Can you work these out from the model? Positions are in its coordinate system, mm. Face numbers are marked on the shaded views. A direction names the side the tool comes from. Coordinates: 2 decimals unless noted, no trailing zeros. Order: outer loops, then holes, each group sorted by start corner. A loop starts at its lowest first (then second) coordinate and runs counter-clockwise, first axis right, second up. Notation, with made-up numbers: M 67.25,-13.75 L 97.25,-13.75 A18 cw 97.25,-7.75 Z; hole C -12,41 d4. An arc over 180 degrees is marked long. Answer as a JSON object with one key per item and string values.
from build123d import *

# Parameters (mm, degrees)
F0_W      = 60
F0_H      = 60
F0_R      = 2.3
F0_R_2    = 19.05
F0_R_3    = 4
F1_DEPTH  = 4.8
F2_DEPTH  = 1.6
F3_DEPTH  = 20.6
F4_R      = 4
F5_W      = 15
F5_H      = 0.5
F6_DEPTH  = 60.001
F7_W      = 37.14
F7_H      = 11.43
F7_H_2    = 37.14
F7_W_2    = 11.43
F8_DEPTH  = 89
F9_R      = 4
F10_R     = 3
F11_R     = 3.25
F12_DEPTH = 14


with BuildPart() as f1:
    # F0 (on Front) → F1 (new body)
    with BuildSketch(Plane.XZ):
        Rectangle(F0_W, F0_H)
        with Locations((-25.1, -25.1)):
            Circle(F0_R, mode=Mode.SUBTRACT)
        with Locations((25.1, -25.1)):
            Circle(F0_R, mode=Mode.SUBTRACT)
        with Locations((-25.1, 25.1)):
            Circle(F0_R, mode=Mode.SUBTRACT)
        Circle(F0_R_2, mode=Mode.SUBTRACT)
        with Locations((25.1, 25.1)):
            Circle(F0_R, mode=Mode.SUBTRACT)
        Circle(F0_R_2)
        Circle(F0_R_3, mode=Mode.SUBTRACT)
        Circle(F0_R_3)
    extrude(amount=-F1_DEPTH)

    # F0 (on Front) → F2 (join)
    with BuildSketch(Plane.XZ):
        Circle(F0_R_2)
        Circle(F0_R_3, mode=Mode.SUBTRACT)
    extrude(amount=F2_DEPTH)

    # F0 (on Front) → F3 (join)
    with BuildSketch(Plane.XZ):
        Circle(F0_R_3)
    extrude(amount=F3_DEPTH)

    # F4
    f4_edges = [f1.edges().sort_by_distance(p)[0] for p in [
        (-30, 2.4, 30),
        (30, 2.4, 30),
        (30, 2.4, -30),
        (-30, 2.4, -30),
    ]]
    fillet(f4_edges, radius=F4_R)

    # F5 (on face) → F6 (cut, through all)
    with BuildSketch(Plane(origin=(-30, 0, 0), x_dir=(0, -1, 0), z_dir=(-1, 0, 0))):
        with Locations((13.1, 3.75)):
            Rectangle(F5_W, F5_H)
    extrude(amount=-F6_DEPTH, mode=Mode.SUBTRACT)

    # F7 (on Front) → F8 (join)
    with BuildSketch(Plane.XZ):
        with Locations((0, 24.285)):
            Rectangle(F7_W, F7_H)
        Rectangle(F7_W, F7_H_2)
        with Locations((-24.285, 0)):
            Rectangle(F7_W_2, F7_H_2)
        with Locations((24.285, 0)):
            Rectangle(F7_W_2, F7_H_2)
        with Locations((0, -24.285)):
            Rectangle(F7_W, F7_H)
    extrude(amount=-F8_DEPTH)

    # F9
    f9_edges = [f1.edges().sort_by_distance(p)[0] for p in [
        (18.57, 46.9, 18.57),
        (-18.57, 46.9, 18.57),
        (-18.57, 46.9, -18.57),
        (18.57, 46.9, -18.57),
    ]]
    fillet(f9_edges, radius=F9_R)

    # F10
    f10_edges = [f1.edges().sort_by_distance(p)[0] for p in [
        (18.57, 46.9, 30),
        (30, 46.9, 18.57),
        (30, 46.9, -18.57),
        (18.57, 46.9, -30),
        (-18.57, 46.9, -30),
        (-30, 46.9, -18.57),
        (-30, 46.9, 18.57),
        (-18.57, 46.9, 30),
    ]]
    fillet(f10_edges, radius=F10_R)

    # F11 (on face) → F12 (join)
    with BuildSketch(Plane(origin=(0, 89, 0), x_dir=(-1, 0, 0), z_dir=(0, 1, 0))):
        Circle(F11_R)
    extrude(amount=F12_DEPTH)


solid = f1.part
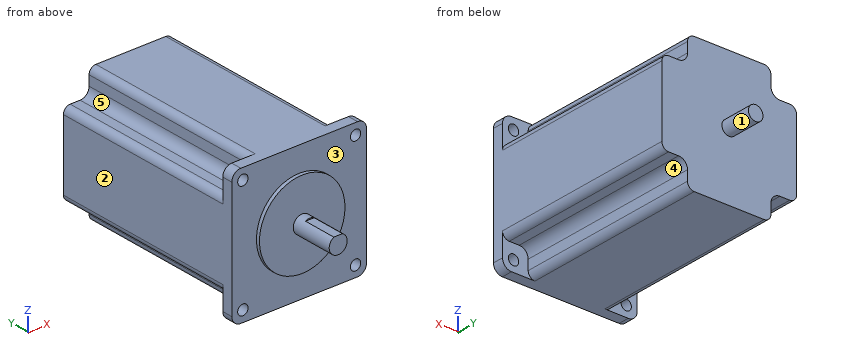
Item 1: I want a section at A-A, the plane x = 0. Write out the boundary of the cut face in (y, z), plus the area to 3 significant figures.
Answers follow:
{"outline": "M -20.6,-4 L -1.6,-4 L -1.6,-19.05 L 0,-19.05 L 0,-30 L 89,-30 L 89,-3.25 L 103,-3.25 L 103,3.25 L 89,3.25 L 89,30 L 0,30 L 0,19.05 L -1.6,19.05 L -1.6,4 L -5.6,4 L -5.6,3.5 L -20.6,3.5 Z", "area": "5,640 mm^2"}
Item 2: I want a section at B-B, the plane y = 53.5. Write out the boundary of the cut face in (x, z), plus the area to 3 significant figures.
Answers follow:
{"outline": "M -30,-15.57 A3 ccw -27,-18.57 L -22.57,-18.57 A4 cw -18.57,-22.57 L -18.57,-27 A3 ccw -15.57,-30 L 15.57,-30 A3 ccw 18.57,-27 L 18.57,-22.57 A4 cw 22.57,-18.57 L 27,-18.57 A3 ccw 30,-15.57 L 30,15.57 A3 ccw 27,18.57 L 22.57,18.57 A4 cw 18.57,22.57 L 18.57,27 A3 ccw 15.57,30 L -15.57,30 A3 ccw -18.57,27 L -18.57,22.57 A4 cw -22.57,18.57 L -27,18.57 A3 ccw -30,15.57 Z", "area": "3,080 mm^2"}
Item 3: Please list where these lines run through material, in increasing order: line 1 (X direction, y = 2, z = -25); line 2 (Y direction, x = -27, z = 0).
Answers follow:
{"line 1": "x = -30 to -27.4, -22.8 to 22.8, 27.4 to 30", "line 2": "y = 0 to 89"}
Item 4: I'm going to push flat-ended pins straight in: pin 1 (1.3 mm diameter, centred on y = 56.5, z = 26, fed in from +X); pin 2 (7.5 mm diameter, centred on x = -25.1, z = 25.1, fed in from -Y); pin 3 (3 mm diameter, centred on x = -20.5, z = -13.5, fed in from +Y). Where does each tip first touch, or does it pass through?
Answers follow:
{"pin 1": "stops at x = 18.57", "pin 2": "stops at y = 0", "pin 3": "stops at y = 89"}
Item 5: Which directions (+Z, -Z, +X, -X, +Y, -Y) give clear straight access to the entire face, cutting with the end or side of a thin tool? Please do the marked faces 1, 2, 3, 4 and 5.
Answers follow:
{"face 1": "+Y", "face 2": "+Z, -Z, -X, +Y, -Y", "face 3": "-Y", "face 4": "-Z, +X, +Y", "face 5": "+Z, -X, +Y"}
